from build123d import *

# Parameters (mm, degrees)
SKETCH1_W           = 37.2
SKETCH1_H           = 63.2
BOSS_EXTRUDE1_DEPTH = 15.5
FILLET1_R           = 2
SHELL1_START        = -16.6
SHELL1_OUTLINE_W    = 13.5
SHELL1_OUTLINE_H    = 59.2
SHELL1_DEPTH        = 33.2
CUT_EXTRUDE1_START  = 9.5
SKETCH2_W           = 37.2
SKETCH2_H           = 61.2
CUT_EXTRUDE1_DEPTH  = 4
SKETCH3_W           = 2.7
SKETCH3_H           = 1
SKETCH3_W_2         = 1
SKETCH3_H_2         = 47.2
SKETCH3_W_3         = 33.2
SKETCH3_H_3         = 1.2
BOSS_EXTRUDE2_DEPTH = 7
SKETCH4_W           = 3.5
SKETCH4_H           = 1
CUT_EXTRUDE2_DEPTH  = 7


# Read off the part's stored shape, not the designer's step: Shell1
with BuildPart() as part:
    # Sketch1 → Boss-Extrude1 (new body)
    with BuildSketch(Plane(origin=(0, 0, 0), x_dir=(1, 0, 0), z_dir=(0, 1, 0))):
        Rectangle(SKETCH1_W, SKETCH1_H)
    extrude(amount=BOSS_EXTRUDE1_DEPTH)

    # Fillet1
    fillet1_edges = [part.edges().sort_by_distance(p)[0] for p in [
        (-18.6, 15.5, 0),
        (0, 15.5, 31.6),
        (18.6, 15.5, 0),
        (0, 0, 31.6),
        (-18.6, 0, 0),
        (0, 0, -31.6),
        (18.6, 0, 0),
        (18.6, 7.75, 31.6),
        (-18.6, 7.75, 31.6),
        (-18.6, 7.75, -31.6),
        (18.6, 7.75, -31.6),
        (0, 15.5, -31.6),
    ]]
    fillet(fillet1_edges, radius=FILLET1_R)

    # Shell1 outline → Shell1 (cut)
    with BuildSketch(Plane.YZ.offset(SHELL1_START)):
        with Locations((8.75, 0)):
            Rectangle(SHELL1_OUTLINE_W, SHELL1_OUTLINE_H)
    extrude(amount=SHELL1_DEPTH, mode=Mode.SUBTRACT)

    # Sketch2 → Cut-Extrude1 (cut)
    with BuildSketch(Plane(origin=(0, 2, 0), x_dir=(1, 0, 0), z_dir=(0, 1, 0)).offset(CUT_EXTRUDE1_START)):
        with Locations((0, -1)):
            Rectangle(SKETCH2_W, SKETCH2_H)
    extrude(amount=CUT_EXTRUDE1_DEPTH, mode=Mode.SUBTRACT)

    # Sketch3 → Boss-Extrude2 (add)
    with BuildSketch(Plane(origin=(0, 2, 0), x_dir=(1, 0, 0), z_dir=(0, 1, 0))):
        with Locations((-15.25, 25.9)):
            Rectangle(SKETCH3_W, SKETCH3_H)
        with Locations((-7.55, 25.9)):
            Rectangle(SKETCH3_W, SKETCH3_H)
        Polygon((-6.2, 29.6), (-6.2, 28.4), (-6.2, 26.4), (-6.2, 25.4), (-6.2, -20.6), (-5.2, -20.6), (-5.2, 26.6), (-5.2, 27.6), (-5.2, 29.6), align=None)
        with Locations((-3.85, 27.1)):
            Rectangle(SKETCH3_W, SKETCH3_H)
        Polygon((8.9, 27.6), (2.5, 27.6), (2.5, 26.6), (5.2, 26.6), (6.2, 26.6), (8.9, 26.6), align=None)
        with Locations((15.25, 27.1)):
            Rectangle(SKETCH3_W, SKETCH3_H)
        with Locations((5.7, 3)):
            Rectangle(SKETCH3_W_2, SKETCH3_H_2)
        with Locations((-15.25, -21.1)):
            Rectangle(SKETCH3_W, SKETCH3_H)
        Polygon((-5.2, -20.6), (-6.2, -20.6), (-8.9, -20.6), (-8.9, -21.6), (-2.5, -21.6), (-2.5, -20.6), align=None)
        Polygon((5.2, -20.6), (2.5, -20.6), (2.5, -21.6), (8.9, -21.6), (8.9, -20.6), (6.2, -20.6), align=None)
        with Locations((15.25, -21.1)):
            Rectangle(SKETCH3_W, SKETCH3_H)
        with Locations((0, -23.1)):
            Rectangle(SKETCH3_W_3, SKETCH3_H)
        with Locations((-15.25, 29)):
            Rectangle(SKETCH3_W, SKETCH3_H_3)
        with Locations((-7.55, 29)):
            Rectangle(SKETCH3_W, SKETCH3_H_3)
    extrude(amount=BOSS_EXTRUDE2_DEPTH)

    # Sketch4 → Cut-Extrude2 (cut)
    with BuildSketch(Plane(origin=(0, 9, 0), x_dir=(1, 0, 0), z_dir=(0, 1, 0))):
        with Locations((-11.4, -23.1)):
            Rectangle(SKETCH4_W, SKETCH4_H)
        with Locations((0, -23.1)):
            Rectangle(SKETCH4_W, SKETCH4_H)
        with Locations((11.4, -23.1)):
            Rectangle(SKETCH4_W, SKETCH4_H)
    extrude(amount=-CUT_EXTRUDE2_DEPTH, mode=Mode.SUBTRACT)


solid = part.part
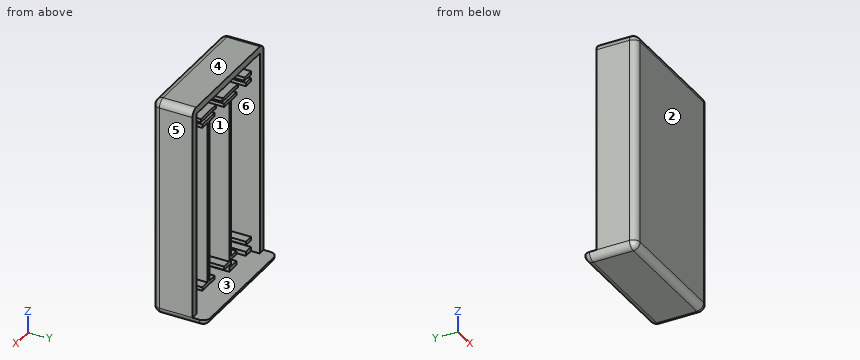
Part model, mm, in its own coordinate system. Face numbers are marked on the shaded views. A direction names the side the tool comes from. Give positions to 0.01 mm unless a question says otherwise; leave off trailing zeros. Write each loop counter-clockwise with the first axis right and the second up, starting at its lowest first coordinate (ties: lowest second). Pieces come first, ordered by that corner, then holes.
1) Pin check, flat tips, straight feed: pin 1 (8 mm diameter, centred on x = 5.5, y = 13.5, fed in from +Z); pin 2 (0.8 mm diameter, centred on x = -15, z = 23, fed in from +Y). Stop position of each tip, or through.
Resolved:
pin 1: stops at z = 31.6
pin 2: stops at y = 9
2) Two-plate mould, pull along Z, no slides. Class the marked faces 3, 4, 5 and 6: released by +Z, released by -Z, zero draft, split by the parting line, or undercut.
Resolved:
face 3: undercut
face 4: released by +Z
face 5: zero draft
face 6: undercut
3) Cut at C-C on z = 14. Write the cut outline in (x, y).
Resolved:
outline: (-18.6, 2) arc R2 ccw to (-16.6, 0) - (16.6, 0) arc R2 ccw to (18.6, 2) - (18.6, 11.5) - (16.6, 11.5) - (16.6, 2) - (6.2, 2) - (6.2, 9) - (5.2, 9) - (5.2, 2) - (-5.2, 2) - (-5.2, 9) - (-6.2, 9) - (-6.2, 2) - (-16.6, 2) - (-16.6, 11.5) - (-18.6, 11.5) - close
4) Cut at B-B on x = 12.5. Write the cut outline in (y, z).
Resolved:
outline: (0, -29.6) arc R2 ccw to (2, -31.6) - (13.5, -31.6) arc R2 ccw to (15.5, -29.6) - (2, -29.6) - (2, 29.6) - (11.5, 29.6) - (11.5, 31.6) - (2, 31.6) arc R2 ccw to (0, 29.6) - close
5) Which spindle directions (+Z, -Z, +X, -X, +Y, -Y) get a long thin tool onto all of the face, cutting with end or side? Do the marked faces 1 and 2. Say none if no direction does.
Resolved:
face 1: +Y
face 2: +Z, -Z, +X, -X, -Y
6) Cut at A-A on y = 3.75. State how many separate pieces and enclosed holes the cut face has, then the cut area to 3 significant figures.
Resolved:
separate pieces: 4
enclosed holes: 1
area: 544 mm2
7) Cut at D-D on x = 4. Write the cut outline in (y, z).
Resolved:
outline: (0, -29.6) arc R2 ccw to (2, -31.6) - (13.5, -31.6) arc R2 ccw to (15.5, -29.6) - (2, -29.6) - (2, -27.6) - (9, -27.6) - (9, -26.6) - (2, -26.6) - (2, 20.6) - (9, 20.6) - (9, 21.6) - (2, 21.6) - (2, 22.6) - (9, 22.6) - (9, 23.6) - (2, 23.6) - (2, 29.6) - (11.5, 29.6) - (11.5, 31.6) - (2, 31.6) arc R2 ccw to (0, 29.6) - close
8) Probe L1, parallel to X at y = 4.5, z = -0.5; L2, parallel to Z at x = -7, y = 3.5; L3, parallel to Z at x = 3.5, y = 6.75. List the from-to ranges inside material, lowest first.
Resolved:
L1: x = -18.6 to -16.6, -6.2 to -5.2, 5.2 to 6.2, 16.6 to 18.6
L2: z = -31.6 to -28.4, -26.4 to -25.4, 20.6 to 21.6, 22.6 to 23.6, 29.6 to 31.6
L3: z = -31.6 to -29.6, -27.6 to -26.6, 20.6 to 21.6, 22.6 to 23.6, 29.6 to 31.6
